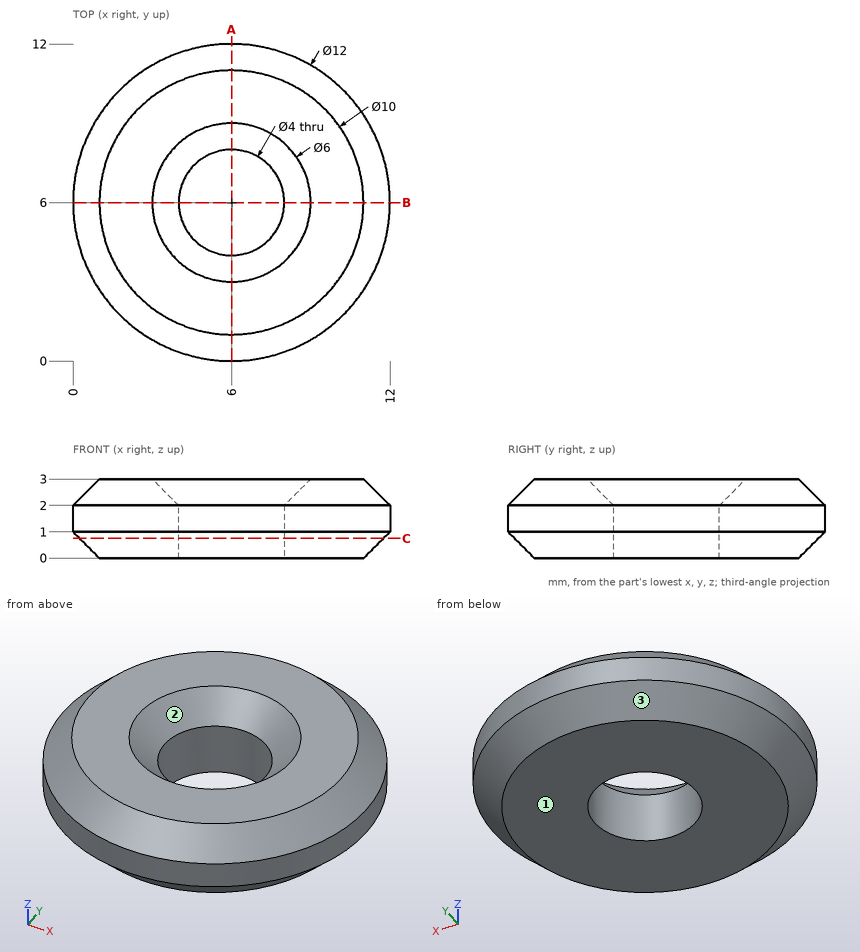
Check sheet for the drawn part. Datum: minimum x, y, z corner. Units: mm. Round coordinates to 2 decimals unless told otherwise and drop trailing zeros. Write each loop counter-clockwise with the first axis right and the second up, starting at its lowest first coordinate (ties: lowest second). Pieces come first, ordered by that corner, then holes. Notation, with made-up numbers: (14, -11.5) - (31, -11.5) arc R36 ccw to (31, 25.5) - close; hole circle Ø11 at (57, -4). An arc over 180 degrees is marked (long way). Write each question's results on one line, items separated by ' | '.
(1) Sectioned sample at C-C, the plane z = 0.75. Enter the section's corners in (x, y), plus the area to 3 significant figures.
Computed:
outline: circle Ø11.5 at (6, 6); hole circle Ø4 at (6, 6) | area: 91.3 mm^2
(2) Sectioned sample at A-A, the plane x = 6. Enter the section's corners in (y, z).
Computed:
outline: (0, 1) - (1, 0) - (4, 0) - (4, 2) - (3, 3) - (1, 3) - (0, 2) - close; (8, 0) - (11, 0) - (12, 1) - (12, 2) - (11, 3) - (9, 3) - (8, 2) - close
(3) Thickness scan on probe 1 along Y at (x, z) = (6, 1.4); probe 2 along Y at (x, z) = (6, 0.65); probe 3 along X at (y, z) = (7, 0.85). Record the ranges inside material, lowest first. Write a range as from..to.
Computed:
probe 1: y = 0..4, 8..12 | probe 2: y = 0.35..4, 8..11.65 | probe 3: x = 0.24..4.27, 7.73..11.76
(4) Draft check along X on the marked faces 1, 2 and 3. Enter one of: pulls with the +X half, pulls with the -X half, needs draft (parallel to the pull), parting line crosses it, or undercut.
Computed:
face 1: needs draft | face 2: undercut | face 3: parting line crosses it
(5) Depth check by flat-ended pin: pin 1 Ø2.5 at (x, y) = (6, 6) entering from -Z. Enter the tip coordinate at first touch or a pass-through.
Computed:
pin 1: passes through
